from build123d import *

# Parameters (mm, degrees)
F0_W     = 5.08
F0_H     = 5.08
F1_DEPTH = 25.4
F2_W     = 2.54
F2_H     = 7.62
F3_DEPTH = 6.35
F4_DEPTH = 12.7
F6_DEPTH = 7.62
F8_DEPTH = 2.54


with BuildPart() as f1:
    # F0 (on Front) → F1 (new body)
    with BuildSketch(Plane.XZ):
        Rectangle(F0_W, F0_H)
    extrude(amount=F1_DEPTH)

    # F2 (on face) → F3 (join)
    with BuildSketch(Plane(origin=(0, 0, -2.54), x_dir=(1, 0, 0), z_dir=(0, 0, -1))):
        with Locations((-1.9143006529, 19.5104427957)):
            Rectangle(F2_W, F2_H)
        with BuildLine():
            Line((-0.6443006529, 15.7004427957), (-3.1843006529, 15.7004427957))
            ThreePointArc((-3.1843006529, 15.7004427957), (-1.9143006529, 14.4304427957), (-0.6443006529, 15.7004427957))
        make_face()
    extrude(amount=F3_DEPTH)

    # F4 (add): a face of the model
    f4_faces = [f1.faces().sort_by_distance(p)[0] for p in [
        (0, 0, 0),
    ]]
    extrude(f4_faces, amount=F4_DEPTH)

    # F5 (on face) → F6 (join)
    with BuildSketch(Plane(origin=(0, 12.7, 0), x_dir=(-1, 0, 0), z_dir=(0, 1, 0))):
        with BuildLine():
            ThreePointArc((0, -2.54), (1.7960512242, -1.7960512242), (2.54, 0))
            ThreePointArc((2.54, 0), (1.7960512242, 1.7960512242), (0, 2.54))
            ThreePointArc((0, 2.54), (-1.7960512242, 1.7960512242), (-2.54, 0))
            ThreePointArc((-2.54, 0), (-1.7960512242, -1.7960512242), (0, -2.54))
        make_face()
    extrude(amount=F6_DEPTH)

    # F7 (on face) → F8 (join)
    with BuildSketch(Plane(origin=(0, 20.32, 0), x_dir=(-1, 0, 0), z_dir=(0, 1, 0))):
        with BuildLine():
            ThreePointArc((0.5929512242, 2.4698195978), (0, 2.6476778516), (-0.5929512242, 2.4698195978))
            ThreePointArc((-0.5929512242, 2.4698195978), (0, 2.54), (0.5929512242, 2.4698195978))
        make_face()
    extrude(amount=-F8_DEPTH)


solid = f1.part
Could you check a few things on this model? Use its own coordinates, in mm. A direction names the side the tool comes from. Give positions to 0.01 mm unless a question says otherwise; leave off trailing zeros. Order: outer loops, then holes, each group sorted by start corner. A loop starts at its lowest first (then second) coordinate and runs counter-clockwise, first axis right, second up. Notation, with made-up numbers: (65.25, 24) - (78.25, 24) arc R18 ccw to (78.25, 44) - close; hole circle Ø10 at (-17.75, -1.5). An arc over 180 degrees is marked (long way). One line per item, written item: value. Start each with the question number.
1. For faces 1 (the face through (-2, 12.7, -2)), 2 (the face through (-2.54, -7, 0)), 3 (the face through (-2, -23.32, -6)), which set-ups out of +Z, -Z, +X, -X, +Y, -Y let a thin tool reach every point of the face, with its end or its side?
2. Imagine slicing it at C-C on x = -1.2. List the corners of the cut face in (y, z) for me, plus the area to 3 significant figures.
3. Imagine slicing it at B-B on y = -15. List the corners of the cut face in (x, z) for me.
4. For P1, Ø1.5, axis at y = -6.5, z = 1, coming from the -X side; P2, Ø3, axis at y = -18, z = -6, coming from the +X side; P3, Ø0.8, axis at x = -1.5, z = -7, coming from the -Y side, each with a flat end and sliding along its axis, tell me the tip position at first contact or that it passes through.
5. If I drill on probe 1 along Z at (x, y) = (1.6, 5); probe 2 along Y at (x, z) = (-2.55, -7.5), over which ranges is the centre line in solid material (lowest first)?
6. Imagine slicing it at D-D on z = -3.75. List the corners of the cut face in (x, y) for me, plus the area to 3 significant figures.
7. Imagine slicing it at A-A on z = 0.75. List the corners of the cut face in (x, y) for me.
Values:
1. face 1: -Z, -X, +Y
1. face 2: +Z, -X, +Y, -Y
1. face 3: -Z, +X, -X, -Y
2. outline: (-25.4, -2.54) - (-23.32, -2.54) - (-23.32, -8.89) - (-14.65, -8.89) - (-14.65, -2.54) - (12.7, -2.54) - (12.7, -2.24) - (20.32, -2.24) - (20.32, 2.24) - (12.7, 2.24) - (12.7, 2.54) - (-25.4, 2.54) - close
2. area: 283 mm²
3. outline: (-2.97, -8.89) - (-0.85, -8.89) - (-0.85, -2.54) - (2.54, -2.54) - (2.54, 2.54) - (-2.54, 2.54) - (-2.54, -2.54) - (-2.97, -2.54) - close
4. P1: x = -2.54
4. P2: x = -0.64
4. P3: y = -23.32
5. probe 1: -2.54 to 2.54
5. probe 2: -23.32 to -14.6
6. outline: (-3.18, -23.32) - (-0.64, -23.32) - (-0.64, -15.7) arc R1.27 ccw to (-3.18, -15.7) - close
6. area: 21.9 mm²
7. outline: (-2.54, -25.4) - (2.54, -25.4) - (2.54, 12.7) - (2.43, 12.7) - (2.43, 20.32) - (-2.43, 20.32) - (-2.43, 12.7) - (-2.54, 12.7) - close
